Geometry: final body of the model. Coordinates: model frame, mm. A direction names the side the tool comes from. Give positions to 0.01 mm unless a question says otherwise; leave off trailing zeros. Write each loop counter-clockwise with the first axis right and the second up, starting at its lowest first coordinate (ties: lowest second). Pieces come first, ordered by that corner, then holes. Notation, with made-up numbers: (32.5, -37) -> (36.5, -37) arc R10 cw to (36.5, -18) -> close; hole circle Ø10 at (46, 4.5). An arc over 180 degrees is marked (long way). Answer as a JSON object with one key per item and string values.
from build123d import *

# Parameters (mm, degrees)
SKETCH1_R           = 3.81
BOSS_EXTRUDE1_DEPTH = 19.05
SKETCH1_3_R         = 3.81
SKETCH1_3_R_2       = 2.159
BOSS_EXTRUDE2_DEPTH = 2.54
SKETCH2_W           = 6.35
SKETCH2_H           = 1.778
CUT_EXTRUDE2_DEPTH  = 58.700024564


with BuildPart() as part:
    # Sketch1 → Boss-Extrude1 (new body)
    with BuildSketch(Plane(origin=(0, 0, 0), x_dir=(1, 0, 0), z_dir=(0, 1, 0))):
        Polygon((-5.944680851, 17.581843972), (-16.104680851, 17.581843972), (-16.104680851, -16.708156028), (-5.944680851, -16.708156028), (-5.944680851, -12.898156028), (0.405319149, -12.898156028), (0.405319149, -16.708156028), (25.805319149, -16.708156028), (25.805319149, -12.898156028), (32.155319149, -12.898156028), (32.155319149, -16.708156028), (42.315319149, -16.708156028), (42.315319149, 17.581843972), (32.155319149, 17.581843972), (32.155319149, 13.771843972), (25.805319149, 13.771843972), (25.805319149, 17.581843972), (16.280319149, 17.581843972), (16.280319149, 4.881843972), (9.930319149, 4.881843972), (9.930319149, 17.581843972), (0.405319149, 17.581843972), (0.405319149, 13.771843972), (-5.944680851, 13.771843972), align=None)
        with Locations(Location((-11.024680851, 12.501843972, 0), (0, 0, 90))):
            Circle(SKETCH1_R, mode=Mode.SUBTRACT)
        with Locations(Location((37.235319149, 12.501843972, 0), (0, 0, 90))):
            Circle(SKETCH1_R, mode=Mode.SUBTRACT)
        with Locations(Location((37.235319149, -11.628156028, 0), (0, 0, 90))):
            Circle(SKETCH1_R, mode=Mode.SUBTRACT)
        with Locations(Location((-11.024680851, -11.628156028, 0), (0, 0, 90))):
            Circle(SKETCH1_R, mode=Mode.SUBTRACT)
    extrude(amount=BOSS_EXTRUDE1_DEPTH)

    # Sketch1_3 → Boss-Extrude2 (add)
    # profile 1 of 4: a face of its own
    with BuildSketch(Plane(origin=(0, 0, 0), x_dir=(1, 0, 0), z_dir=(0, 1, 0))):
        with Locations(Location((-11.024680851, 12.501843972, 0), (0, 0, 90))):
            Circle(SKETCH1_3_R)
        with Locations(Location((-11.024680851, 12.501843972, 0), (0, 0, 270))):
            Circle(SKETCH1_3_R_2, mode=Mode.SUBTRACT)
    # profile 2 of 4: a face of its own
    with BuildSketch(Plane(origin=(0, 0, 0), x_dir=(1, 0, 0), z_dir=(0, 1, 0))):
        with Locations(Location((-11.024680851, -11.628156028, 0), (0, 0, 90))):
            Circle(SKETCH1_3_R)
        with Locations(Location((-11.024680851, -11.628156028, 0), (0, 0, 270))):
            Circle(SKETCH1_3_R_2, mode=Mode.SUBTRACT)
    # profile 3 of 4: a face of its own
    with BuildSketch(Plane(origin=(0, 0, 0), x_dir=(1, 0, 0), z_dir=(0, 1, 0))):
        with Locations(Location((37.235319149, 12.501843972, 0), (0, 0, 90))):
            Circle(SKETCH1_3_R)
        with Locations(Location((37.235319149, 12.501843972, 0), (0, 0, 270))):
            Circle(SKETCH1_3_R_2, mode=Mode.SUBTRACT)
    # profile 4 of 4: a face of its own
    with BuildSketch(Plane(origin=(0, 0, 0), x_dir=(1, 0, 0), z_dir=(0, 1, 0))):
        with Locations(Location((37.235319149, -11.628156028, 0), (0, 0, 90))):
            Circle(SKETCH1_3_R)
        with Locations(Location((37.235319149, -11.628156028, 0), (0, 0, 270))):
            Circle(SKETCH1_3_R_2, mode=Mode.SUBTRACT)
    extrude(amount=BOSS_EXTRUDE2_DEPTH)

    # Sketch2 → Cut-Extrude2 (cut, through all)
    with BuildSketch(Plane.XY.offset(16.708156028)):
        with Locations((-2.769680851, 0.889)):
            Rectangle(SKETCH2_W, SKETCH2_H)
        with Locations((28.980319149, 0.889)):
            Rectangle(SKETCH2_W, SKETCH2_H)
    extrude(amount=-CUT_EXTRUDE2_DEPTH, mode=Mode.SUBTRACT)


solid = part.part
Q1. Cut plane B-B (y = 18). Return the cut outline in (x, z).
Values:
{"outline": "(-16.1, -17.58) -> (-5.94, -17.58) -> (-5.94, -13.77) -> (0.41, -13.77) -> (0.41, -17.58) -> (9.93, -17.58) -> (9.93, -4.88) -> (16.28, -4.88) -> (16.28, -17.58) -> (25.81, -17.58) -> (25.81, -13.77) -> (32.16, -13.77) -> (32.16, -17.58) -> (42.32, -17.58) -> (42.32, 16.71) -> (32.16, 16.71) -> (32.16, 12.9) -> (25.81, 12.9) -> (25.81, 16.71) -> (0.41, 16.71) -> (0.41, 12.9) -> (-5.94, 12.9) -> (-5.94, 16.71) -> (-16.1, 16.71) -> close; hole circle Ø7.62 at (-11.02, -12.5); hole circle Ø7.62 at (-11.02, 11.63); hole circle Ø7.62 at (37.24, -12.5); hole circle Ø7.62 at (37.24, 11.63)"}
Q2. First-contact query: P1, Ø2, axis at x = 31, z = -0.5, coming from the -Y side; P2, Ø3, axis at x = 29, y = 9, coming from the +Z side; P3, Ø5, axis at x = 30, y = 11, coming from the -Z side; P4, Ø2.5, axis at x = -9.5, z = -13.5, coming from the +Y side. Flat tips, straight axial feed; report the tip coordinate or a pass-through.
Values:
{"P1": "y = 1.78", "P2": "z = 12.9", "P3": "z = -17.58", "P4": "y = 2.54"}
Q3. Mould query, pull axis X, two halves, no side actions, for faces 1 (the flat face through (-11, 0, 0)), 2 (the flat face through (-16.105, 9, -1)), 3 (the flat face through (-3, 1.778, 0)). Classes: pulls with the +X half, pulls with the -X half, needs draft (parallel to the pull), parting line crosses it, or undercut.
Values:
{"face 1": "needs draft", "face 2": "pulls with the -X half", "face 3": "undercut"}
Q4. Cut plane A-A (z = 1). Return the cut outline in (x, y), and give its area (3 significant figures).
Values:
{"outline": "(-16.1, 0) -> (-5.94, 0) -> (-5.94, 1.78) -> (0.41, 1.78) -> (0.41, 0) -> (25.81, 0) -> (25.81, 1.78) -> (32.16, 1.78) -> (32.16, 0) -> (42.32, 0) -> (42.32, 19.05) -> (-16.1, 19.05) -> close", "area": "1,090 mm²"}
Q5. Set-up query: faces 4 (the flat face through (-3, 10, -13.772)), 5 (the flat face through (37, 9, -17.582)), 6 (the flat face through (32.155, 1, 1)), 7 (the cylindrical face through (33.458, 10.679, 12.124)). Return all of +Z, -Z, +X, -X, +Y, -Y with unobstructed straight access to the full face (end or side cutting, diameter ignored); none if empty.
Values:
{"face 4": "-Z, +Y, -Y", "face 5": "-Z, +X, -X, +Y, -Y", "face 6": "-Y", "face 7": "+Y"}
Q6. Material intervals for L1, parallel to X at y = 1, z = -5; L2, parallel to X at y = 6.75, z = -8.5; L3, parallel to Z at x = -11.5, y = 15, sorted ascending. Write a range as from..to.
Values:
{"L1": "-16.1..-5.94, 0.41..9.93, 16.28..25.81, 32.16..42.32", "L2": "-16.1..9.93, 16.28..42.32", "L3": "-17.58..-16.28, -8.72..7.85, 15.41..16.71"}
Q7. Cut plane C-C (x = 34). Return the cut outline in (y, z), and give its area (3 significant figures).
Values:
{"outline": "(0, -17.58) -> (19.05, -17.58) -> (19.05, -14.51) -> (2.54, -14.51) -> (2.54, -10.49) -> (19.05, -10.49) -> (19.05, 9.62) -> (2.54, 9.62) -> (2.54, 13.64) -> (19.05, 13.64) -> (19.05, 16.71) -> (0, 16.71) -> close", "area": "520 mm²"}
